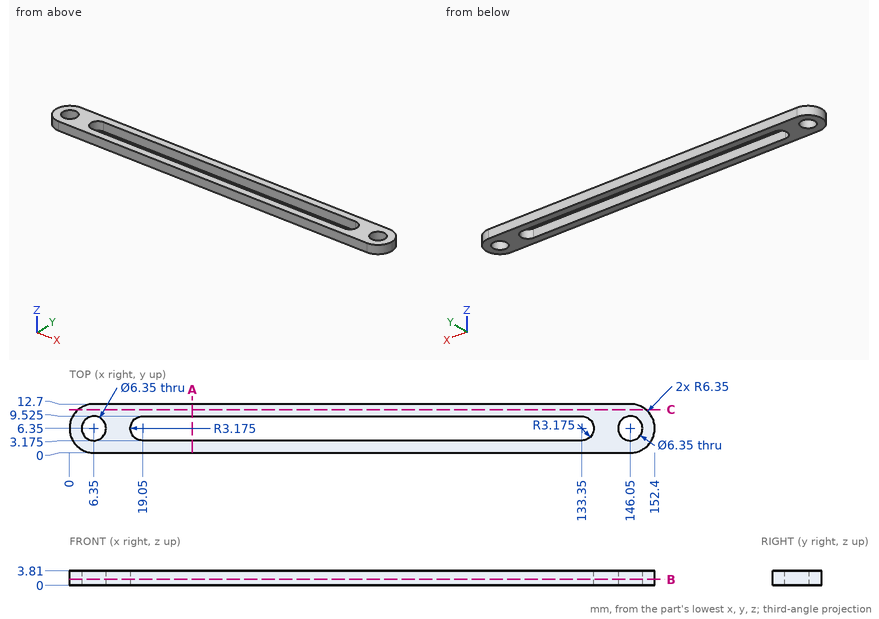
The figure shows three views and two pictorial views of one solid part (mm, origin at its lowest corner). Answer the questions. Give positions to 0.01 mm unless a question says otherwise; leave off trailing zeros. Order: outer loops, then holes, each group sorted by start corner. A loop starts at its lowest first (then second) coordinate and runs counter-clockwise, first axis right, second up. Notation, with made-up numbers: (29.25, 58) - (60.25, 58) arc R27 cw to (60.25, 87) - close; hole circle Ø11 at (43.5, -2). An arc over 180 degrees is marked (long way). Answer as CSV lines item,"result".
Q1. A cutting plane is placed at A-A, the plane x = 32. Determine the outline of the cut face in (y, z) (3 decimals), and give its area (3 significant figures).
Answer key:
outline,"(0, 0) - (3.175, 0) - (3.175, 3.81) - (0, 3.81) - close; (9.525, 0) - (12.7, 0) - (12.7, 3.81) - (9.525, 3.81) - close"
area,"24.2 mm^2"
Q2. Each of these flat-tipped pins is pushed along its axis until it touches: pin 1 Ø4 at (x, y) = (52.5, 5.5) entering from +Z; pin 2 Ø7.5 at (x, y) = (146.05, 6.35) entering from -Z. Where does it stop, or does it pass through?
Answer key:
pin 1,"passes through"
pin 2,"stops at z = 0"
Q3. A cutting plane is placed at B-B, the plane z = 1.55. Determine the outline of the cut face in (x, y) (3 decimals).
Answer key:
outline,"(6.35, 0) - (146.05, 0) arc R6.35 ccw to (146.05, 12.7) - (6.35, 12.7) arc R6.35 ccw to start; hole circle Ø6.35 at (6.35, 6.35); hole (19.05, 3.175) - (133.35, 3.175) arc R3.175 ccw to (133.35, 9.525) - (19.05, 9.525) arc R3.175 ccw to start; hole circle Ø6.35 at (146.05, 6.35)"
Q4. A cutting plane is placed at C-C, the plane y = 11.25. Determine the outline of the cut face in (x, z).
Answer key:
outline,"(2.31, 0) - (150.09, 0) - (150.09, 3.81) - (2.31, 3.81) - close"
Q5. Straight lines are drawn through the part: L1, parallel to Y at x = 45, z = 1.8 (3 decimals); L2, parallel to X at y = 7.5, z = 2.6 (3 decimals); L3, parallel to X at y = 7.75, z = 3.5. For each, find the intervals that lie inside material, in ascending order.
Answer key:
L1,"y = 0 to 3.175, 9.525 to 12.7"
L2,"x = 0.105 to 3.391, 9.309 to 16.091, 136.309 to 143.091, 149.009 to 152.295"
L3,"x = 0.16 to 3.5, 9.2 to 16.2, 136.2 to 143.2, 148.9 to 152.24"
